```python
from build123d import *

# Parameters (mm, degrees)
SKETCH1_R           = 0.9525
BOSS_EXTRUDE1_DEPTH = 1.27
FILLET1_R           = 1.5875


with BuildPart() as part:
    # Sketch1 → Boss-Extrude1 (new body)
    with BuildSketch(Plane.XY):
        with BuildLine():
            Line((-1.27, -3.793560366), (-1.27, -1.054941231))
            ThreePointArc((-1.27, -1.054941231), (0, 1.651), (1.27, -1.054941231))
            Line((1.27, -1.054941231), (1.27, -3.793560366))
            ThreePointArc((1.27, -3.793560366), (3.974472125, -0.455600239), (2.0955, 3.407767598))
            Line((2.0955, 3.407767598), (2.0955, 4.7625))
            ThreePointArc((2.0955, 4.7625), (0, 6.858), (-2.0955, 4.7625))
            Line((-2.0955, 4.7625), (-2.0955, 3.407767598))
            ThreePointArc((-2.0955, 3.407767598), (-3.974472125, -0.455600239), (-1.27, -3.793560366))
        make_face()
        with Locations((0, 4.7625)):
            Circle(SKETCH1_R, mode=Mode.SUBTRACT)
    extrude(amount=BOSS_EXTRUDE1_DEPTH)

    # Fillet1
    fillet1_edges = [part.edges().sort_by_distance(p)[0] for p in [
        (-2.0955, 3.407767598, 0.635),
        (2.0955, 3.407767598, 0.635),
    ]]
    fillet(fillet1_edges, radius=FILLET1_R)


solid = part.part
```
Here's how the part is built. I have some questions about the finished solid (model axes, mm). A direction names the side the tool comes from. Coordinates: 2 decimals unless noted, no trailing zeros. Write each loop counter-clockwise with the first axis right and the second up, starting at its lowest first coordinate (ties: lowest second). Pieces come first, ordered by that corner, then holes. Notation, with made-up numbers: (36, 40) -> (88, 40) arc R5 cw to (88, 49) -> close; hole circle Ø4 at (-36, 17). An arc over 180 degrees is marked (long way). Use a Markdown table: item, result. Add a question column.
(1) Please list where these lines run through material, in increasing order: line 1 (Y direction, x = 0, z = 0.5) (3 decimals); line 2 (X direction, y = 0, z = 0.7); line 3 (X direction, y = 1, z = 1).
(2) If we section it at D-D, the plane x = -3: Write out the boundary of the cut face in (y, z), and give its area (3 significant figures).
(3) I'm going to push a flat-ended pin straight in: P1, Ø0.6, axis at y = 4.5, z = 0.5, coming from the -X side. Where does the tip first touch, or does it pass through?
(4) If we section it at C-C, the plane x = 0: Write out the boundary of the cut face in (y, z) (3 decimals).
(5) If we section it at B-B, the plane z = 0.3: Write out the boundary of the cut face in (x, y) (1 decimal), and give its area (3 significant figures).
(6) We'd pull the mould along Y, two halves only. Please class faces 3 (the cylindrical face through (-0.124, 5.707, 0.626)), 4 (the cylindrical face through (0.046, 6.857, 0.626)), 5 (the cylindrical face through (-3.933, -0.73, 0.626)): +Y half, -Y half, draft (parallel to the pull), parting line (faces both ways), or undercut.
(7) If we section it at A-A, the plane y = 0: Write out the boundary of the cut face in (x, z).
(8) For faces 1 (the cylindrical face through (-2.24, 3.54, 0.64)), 2 (the flat face through (-1.27, -2, 1)), which set-ups out of +Z, -Z, +X, -X, +Y, -Y let a thin tool reach every point of the face, with its end or its side?
Outcome:
| question | item | result |
|---|---|---|
| 1 | line 1 | y = 1.651 to 3.81, 5.715 to 6.858 |
| 1 | line 2 | x = -4 to -1.65, 1.65 to 4 |
| 1 | line 3 | x = -3.87 to -1.31, 1.31 to 3.87 |
| 2 | outline | (-2.65, 0) -> (2.65, 0) -> (2.65, 1.27) -> (-2.65, 1.27) -> close |
| 2 | area | 6.72 mm^2 |
| 3 | P1 | stops at x = -2.1 |
| 4 | outline | (1.651, 0) -> (3.81, 0) -> (3.81, 1.27) -> (1.651, 1.27) -> close; (5.715, 0) -> (6.858, 0) -> (6.858, 1.27) -> (5.715, 1.27) -> close |
| 5 | outline | (-2.6, 3) arc R4 ccw to (-1.3, -3.8) -> (-1.3, -1.1) arc R1.7 cw (long way) to (1.3, -1.1) -> (1.3, -3.8) arc R4 ccw to (2.6, 3) arc R1.6 cw to (2.1, 4.2) -> (2.1, 4.8) arc R2.1 ccw to (-2.1, 4.8) -> (-2.1, 4.2) arc R1.6 cw to start; hole circle Ø1.9 at (0, 4.8) |
| 5 | area | 43.7 mm^2 |
| 6 | face 3 | undercut |
| 6 | face 4 | +Y half |
| 6 | face 5 | parting line |
| 7 | outline | (-4, 0) -> (-1.65, 0) -> (-1.65, 1.27) -> (-4, 1.27) -> close; (1.65, 0) -> (4, 0) -> (4, 1.27) -> (1.65, 1.27) -> close |
| 8 | face 1 | +Z, -Z, -X, +Y |
| 8 | face 2 | +Z, -Z, -Y |
